Geometry: final body of the model. Coordinates: model frame, mm. Coordinates: 2 decimals unless noted, no trailing zeros. Order: outer loops, then holes, each group sorted by start corner. A loop starts at its lowest first (then second) coordinate and runs counter-clockwise, first axis right, second up. Notation, with made-up numbers: M 26,-1 L 32,-1 A33 cw 32,33 Z; hole C 76,62 d9. An arc over 180 degrees is marked long. Write item = value, one per line.
from build123d import *

# Parameters (mm, degrees)
F3_R = 1


# Not quite as in the source:
# - a fillet or chamfer that OpenCascade refuses, or shapes differently, is made with other operations: its cross-section is extruded or revolved along the edge and cut away or added


with BuildPart() as f1:
    # F0 (on Front) → F1 (revolve)
    with BuildSketch(Plane.XZ):
        with BuildLine():
            Line((-11.5, 0), (0, 0))
            Line((0, 0), (0, 125.5))
            Line((0, 125.5), (-11.5, 125.5))
            Line((-11.5, 125.5), (-11.5, 111.1))
            ThreePointArc((-11.5, 111.1), (-11.4175796144, 111.0506064835), (-11.3358983849, 111))
            Line((-11.3358983849, 111), (-8.3, 111))
            Line((-8.3, 111), (-8.3, 105.5))
            Line((-8.3, 105.5), (-8.3, 100))
            Line((-8.3, 100), (-11.3358983849, 100))
            ThreePointArc((-11.3358983849, 100), (-11.4175796144, 99.9493935165), (-11.5, 99.9))
            Line((-11.5, 99.9), (-11.5, 0))
        make_face()
    revolve(axis=Axis((0, 0, 62.75), (0, 0, 1)))

    # F2: fillet of radius 6.5 on 3 edges, made by hand

    # F2_s1 → F2_t2 (revolve, cut)
    with BuildSketch(Plane.XZ):
        with BuildLine():
            ThreePointArc((-11.5, 119), (-9.5961940777, 123.5961940777), (-5, 125.5))
            Line((-5, 125.5), (-11.5, 125.5))
            Line((-11.5, 125.5), (-11.5, 119))
        make_face()
    revolve(axis=Axis((0, 0, 125.5), (0, 0, 1)), mode=Mode.SUBTRACT)

    # F2_s3 → F2_t4 (revolve)
    with BuildSketch(Plane.XZ):
        with BuildLine():
            ThreePointArc((-8.3, 105.5), (-9.1093646884, 108.6411255548), (-11.3358983849, 111))
            Line((-11.3358983849, 111), (-8.3, 111))
            Line((-8.3, 111), (-8.3, 105.5))
        make_face()
    revolve(axis=Axis((0, 0, 111), (0, 0, 1)))

    # F2_s5 → F2_t6 (revolve)
    with BuildSketch(Plane.XZ):
        with BuildLine():
            ThreePointArc((-11.3358983849, 100), (-9.1093646884, 102.3588744452), (-8.3, 105.5))
            Line((-8.3, 105.5), (-8.3, 100))
            Line((-8.3, 100), (-11.3358983849, 100))
        make_face()
    revolve(axis=Axis((0, 0, 100), (0, 0, 1)))

    # F3
    f3_edges = [f1.edges().sort_by_distance(p)[0] for p in [
        (11.5, 0, 111.1),
        (11.5, 0, 99.9),
    ]]
    fillet(f3_edges, radius=F3_R)


solid = f1.part
1) Line query: L1, parallel to X at y = -0.5, z = 39.5; L2, parallel to Z at x = -5, y = 9.5; L3, parallel to Z at x = 4.5, y = 9.25. Output: solid intervals per line, ascending.
Numbers:
L1 = -11.49 to 11.49
L2 = 0 to 100.43, 110.57 to 122.06
L3 = 0 to 100.82, 110.18 to 122.78
2) Pin query (flat end, axial travel): pin 1 (4 mm diameter, centred on y = -5.5, z = 87.5, fed in from -X); pin 2 (4 mm diameter, centred on y = -7.5, z = 105.5, fed in from +X); pin 3 (8 mm diameter, centred on x = 8.5, y = -3.5, fed in from +Z); pin 4 (12 mm diameter, centred on y = -5, z = 51.5, fed in from +X). Return the tip coordinate at first contact, or that it passes through.
Numbers:
pin_1 = -10.95
pin_2 = 6.22
pin_3 = 125.5
pin_4 = 11.5
3) Section A-A, the plane z = 61. Return loops of the section in (x, y), and give its area (3 significant figures).
Numbers:
outline = C 0,0 d23
area = 415 mm²
